```python
from build123d import *

# Parameters (mm, degrees)
BOSS_EXTRUDE1_DEPTH = 5
CUT_EXTRUDE1_DEPTH  = 5
FILLET1_R           = 2
CONG_1_R            = 5


with BuildPart() as part:
    # Sketch1 → Boss-Extrude1 (new body)
    with BuildSketch(Plane.XY):
        Polygon((-75.813253012, 35), (254.186746988, 35), (254.186746988, 20), (264.186746988, 20), (264.186746988, 10), (254.186746988, 10), (254.186746988, -10), (264.186746988, -10), (264.186746988, -20), (254.186746988, -20), (254.186746988, -35), (-75.813253012, -35), (-75.813253012, -20), (-85.813253012, -20), (-85.813253012, -10), (-75.813253012, -10), (-75.813253012, 10), (-85.813253012, 10), (-85.813253012, 20), (-75.813253012, 20), align=None)
    extrude(amount=BOSS_EXTRUDE1_DEPTH)

    # Sketch2 → Cut-Extrude1 (cut)
    with BuildSketch(Plane.XY.offset(5)):
        with BuildLine():
            Line((-53.813253012, 35), (-47.813253012, 35))
            Line((-47.813253012, 35), (-49.063253012, 20))
            ThreePointArc((-49.063253012, 20), (-50.813253012, 18.25), (-52.563253012, 20))
            Line((-52.563253012, 20), (-53.813253012, 35))
        make_face()
        with BuildLine():
            Line((-13.813253012, 35), (-7.813253012, 35))
            Line((-7.813253012, 35), (-9.063253012, 20))
            ThreePointArc((-9.063253012, 20), (-10.813253012, 18.25), (-12.563253012, 20))
            Line((-12.563253012, 20), (-13.813253012, 35))
        make_face()
        with BuildLine():
            Line((26.186746988, 35), (32.186746988, 35))
            Line((32.186746988, 35), (30.936746988, 20))
            ThreePointArc((30.936746988, 20), (29.186746988, 18.25), (27.436746988, 20))
            Line((27.436746988, 20), (26.186746988, 35))
        make_face()
        with BuildLine():
            Line((66.186746988, 35), (72.186746988, 35))
            Line((72.186746988, 35), (70.936746988, 20))
            ThreePointArc((70.936746988, 20), (69.186746988, 18.25), (67.436746988, 20))
            Line((67.436746988, 20), (66.186746988, 35))
        make_face()
        with BuildLine():
            Line((106.186746988, 35), (112.186746988, 35))
            Line((112.186746988, 35), (110.936746988, 20))
            ThreePointArc((110.936746988, 20), (109.186746988, 18.25), (107.436746988, 20))
            Line((107.436746988, 20), (106.186746988, 35))
        make_face()
        with BuildLine():
            Line((146.186746988, 35), (152.186746988, 35))
            Line((152.186746988, 35), (150.936746988, 20))
            ThreePointArc((150.936746988, 20), (149.186746988, 18.25), (147.436746988, 20))
            Line((147.436746988, 20), (146.186746988, 35))
        make_face()
        with BuildLine():
            Line((186.186746988, 35), (192.186746988, 35))
            Line((192.186746988, 35), (190.936746988, 20))
            ThreePointArc((190.936746988, 20), (189.186746988, 18.25), (187.436746988, 20))
            Line((187.436746988, 20), (186.186746988, 35))
        make_face()
        with BuildLine():
            Line((226.186746988, 35), (232.186746988, 35))
            Line((232.186746988, 35), (230.936746988, 20))
            ThreePointArc((230.936746988, 20), (229.186746988, 18.25), (227.436746988, 20))
            Line((227.436746988, 20), (226.186746988, 35))
        make_face()
        with BuildLine():
            Line((232.186746988, -35), (230.936746988, -20))
            ThreePointArc((230.936746988, -20), (229.186746988, -18.25), (227.436746988, -20))
            Line((227.436746988, -20), (226.186746988, -35))
            Line((226.186746988, -35), (232.186746988, -35))
        make_face()
        with BuildLine():
            Line((192.186746988, -35), (190.936746988, -20))
            ThreePointArc((190.936746988, -20), (189.186746988, -18.25), (187.436746988, -20))
            Line((187.436746988, -20), (186.186746988, -35))
            Line((186.186746988, -35), (192.186746988, -35))
        make_face()
        with BuildLine():
            Line((152.186746988, -35), (150.936746988, -20))
            ThreePointArc((150.936746988, -20), (149.186746988, -18.25), (147.436746988, -20))
            Line((147.436746988, -20), (146.186746988, -35))
            Line((146.186746988, -35), (152.186746988, -35))
        make_face()
        with BuildLine():
            Line((112.186746988, -35), (110.936746988, -20))
            ThreePointArc((110.936746988, -20), (109.186746988, -18.25), (107.436746988, -20))
            Line((107.436746988, -20), (106.186746988, -35))
            Line((106.186746988, -35), (112.186746988, -35))
        make_face()
        with BuildLine():
            Line((72.186746988, -35), (70.936746988, -20))
            ThreePointArc((70.936746988, -20), (69.186746988, -18.25), (67.436746988, -20))
            Line((67.436746988, -20), (66.186746988, -35))
            Line((66.186746988, -35), (72.186746988, -35))
        make_face()
        with BuildLine():
            Line((32.186746988, -35), (30.936746988, -20))
            ThreePointArc((30.936746988, -20), (29.186746988, -18.25), (27.436746988, -20))
            Line((27.436746988, -20), (26.186746988, -35))
            Line((26.186746988, -35), (32.186746988, -35))
        make_face()
        with BuildLine():
            Line((-7.813253012, -35), (-9.063253012, -20))
            ThreePointArc((-9.063253012, -20), (-10.813253012, -18.25), (-12.563253012, -20))
            Line((-12.563253012, -20), (-13.813253012, -35))
            Line((-13.813253012, -35), (-7.813253012, -35))
        make_face()
        with BuildLine():
            Line((-47.813253012, -35), (-49.063253012, -20))
            ThreePointArc((-49.063253012, -20), (-50.813253012, -18.25), (-52.563253012, -20))
            Line((-52.563253012, -20), (-53.813253012, -35))
            Line((-53.813253012, -35), (-47.813253012, -35))
        make_face()
    extrude(amount=-CUT_EXTRUDE1_DEPTH, mode=Mode.SUBTRACT)

    # Fillet1
    fillet1_edges = [part.edges().sort_by_distance(p)[0] for p in [
        (-13.813253012, 35, 2.5),
        (-7.813253012, 35, 2.5),
        (26.186746988, 35, 2.5),
        (32.186746988, 35, 2.5),
        (66.186746988, 35, 2.5),
        (72.186746988, 35, 2.5),
        (106.186746988, 35, 2.5),
        (112.186746988, 35, 2.5),
        (146.186746988, 35, 2.5),
        (152.186746988, 35, 2.5),
        (186.186746988, 35, 2.5),
        (192.186746988, 35, 2.5),
        (226.186746988, 35, 2.5),
        (232.186746988, 35, 2.5),
        (232.186746988, -35, 2.5),
        (226.186746988, -35, 2.5),
        (192.186746988, -35, 2.5),
        (186.186746988, -35, 2.5),
        (152.186746988, -35, 2.5),
        (146.186746988, -35, 2.5),
        (112.186746988, -35, 2.5),
        (106.186746988, -35, 2.5),
        (72.186746988, -35, 2.5),
        (66.186746988, -35, 2.5),
        (32.186746988, -35, 2.5),
        (26.186746988, -35, 2.5),
        (-7.813253012, -35, 2.5),
        (-13.813253012, -35, 2.5),
        (-47.813253012, -35, 2.5),
        (-53.813253012, -35, 2.5),
        (-53.813253012, 35, 2.5),
        (-47.813253012, 35, 2.5),
    ]]
    fillet(fillet1_edges, radius=FILLET1_R)

    # Congé1
    cong_1_edges = [part.edges().sort_by_distance(p)[0] for p in [
        (-75.813253012, 35, 2.5),
        (254.186746988, 35, 2.5),
        (254.186746988, -35, 2.5),
        (-75.813253012, -35, 2.5),
    ]]
    fillet(cong_1_edges, radius=CONG_1_R)


solid = part.part
```
Read the model definition and answer for the solid it produces. Units are mm, in the model's axes. Give positions to 0.01 mm unless a question says otherwise; leave off trailing zeros. Write each loop counter-clockwise with the first axis right and the second up, starting at its lowest first coordinate (ties: lowest second). Pieces come first, ordered by that corner, then holes. Notation, with made-up numbers: (34.5, 5.25) - (47.5, 5.25) arc R15 ccw to (47.5, 33.25) - close; hole circle Ø5 at (-29, 46.25). An arc over 180 degrees is marked (long way). Write item = value, one per line. Start each with the question number.
Item 1: Find section A-A (y = 0.5). Give the vertices of the cut face in (x, z), then the cut area to 3 significant figures.
Item 2: Each of these flat-tipped pins is pushed along its axis until it touches: P1, Ø1.5, axis at y = -1, z = 3, coming from the +X side; P2, Ø1.5, axis at x = -79, z = 3, coming from the +Y side; P3, Ø2.5, axis at y = 23, z = 3, coming from the -X side. Where does it stop, or does it pass through?
Item 3: Find the intervals of material crossed by probe 1 along X at (y, z) = (-2, 1.4); probe 2 along Y at (x, z) = (-47.5, 4.4), in increasing order. Write a range as [from, to].
Response:
q1.outline = (-75.81, 0) - (254.19, 0) - (254.19, 5) - (-75.81, 5) - close
q1.area = 1,650 mm²
q2.P1 = 254.19
q2.P2 = 20
q2.P3 = -75.81
q3.probe_1 = [-75.81, 254.19]
q3.probe_2 = [-34.29, 34.29]
